Job drawing, mm, ordinate dimensions from the low corner. One solid piece. Round coordinates to 2 decimals unless told otherwise and drop trailing zeros. Loops run counter-clockwise (first coordinate to the right, second up) from the corner with the lowest first, then second, coordinate; pieces in that order, holes last.
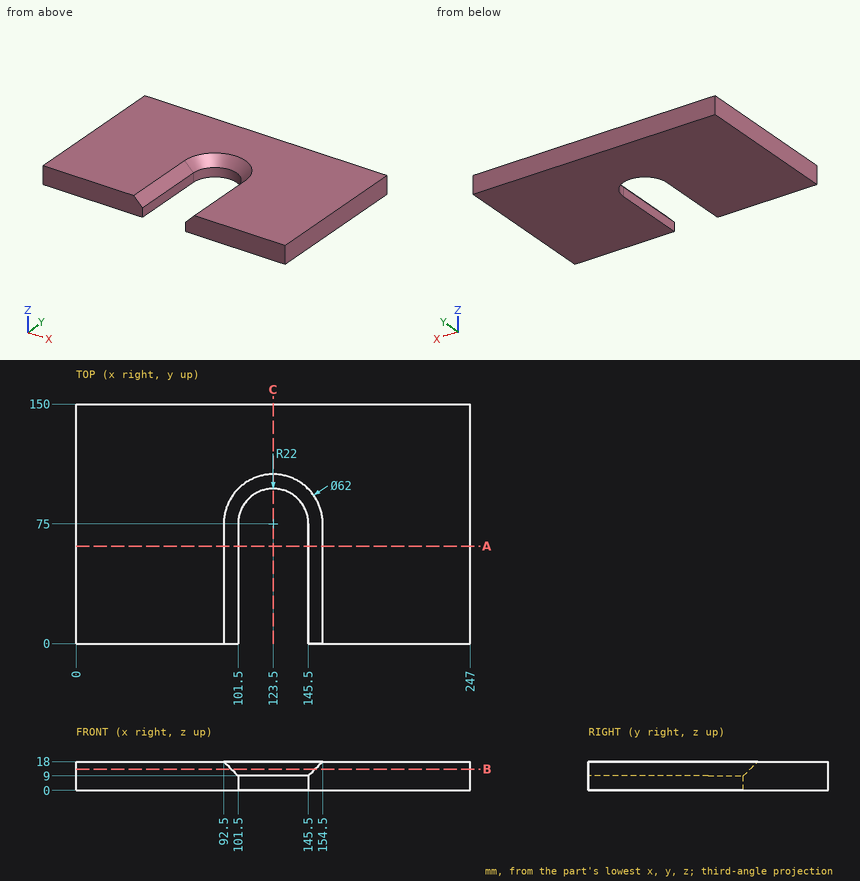
(1) Slice it at A-A on y = 61. List the corners of the cut face in (x, z), plus the area to 3 significant figures.
Responses:
outline: (0, 0) - (101.5, 0) - (101.5, 9) - (92.5, 18) - (0, 18) - close; (145.5, 0) - (247, 0) - (247, 18) - (154.5, 18) - (145.5, 9) - close
area: 3,570 mm2
(2) Probe line 1 (X direction, y = 60, z = 4); line 2 (X direction, y = 28, z = 16.25); line 3 (Y direction, x = 123, z = 6). List the from-to ranges inside material, lowest first.
Responses:
line 1: x = 0 to 101.5, 145.5 to 247
line 2: x = 0 to 94.25, 152.75 to 247
line 3: y = 96.99 to 150
(3) Slice it at C-C on x = 123.5. List the corners of the cut face in (y, z).
Responses:
outline: (97, 0) - (150, 0) - (150, 18) - (106, 18) - (97, 9) - close
(4) Slice it at B-B on z = 13.25. List the corners of the cut face in (x, y), plus the area to 3 significant figures.
Responses:
outline: (0, 0) - (97.25, 0) - (97.25, 75) arc R26.25 cw to (149.75, 75) - (149.75, 0) - (247, 0) - (247, 150) - (0, 150) - close
area: 32,000 mm2
(5) Pin check, flat tips, straight feed: P1, Ø1, axis at y = 92.5, z = 2.5, coming from the -X side; P2, Ø5, axis at x = 107.5, z = 6.5, coming from the -Y side. Stop position of each tip, or through.
Responses:
P1: stops at x = 0
P2: stops at y = 86.91
